```python
from build123d import *

# Parameters (mm, degrees)
ESQUISSE1_W             = 45
ESQUISSE1_H             = 25.2
BOSS_EXTRU_1_DEPTH      = 55
ENL_V_MAT_EXTRU_1_DEPTH = 15.2
ESQUISSE4_W             = 2
ESQUISSE4_H             = 11.757289378
ESQUISSE4_H_2           = 8.71932614
BOSS_EXTRU_2_DEPTH      = 15.2
BOSS_EXTRU_3_DEPTH      = 15.2
CONG_2_R                = 1
CONG_5_R                = 1
CONG_10_R               = 1


with BuildPart() as part:
    # Esquisse1 → Boss.-Extru.1 (new body)
    with BuildSketch(Plane.XY):
        with Locations((0, 2)):
            Rectangle(ESQUISSE1_W, ESQUISSE1_H)
        with BuildLine():
            Line((-4, 3), (-4, -3))
            ThreePointArc((-4, -3), (-6, -5), (-8, -3))
            Line((-8, -3), (-8, 3))
            ThreePointArc((-8, 3), (-6, 5), (-4, 3))
        make_face(mode=Mode.SUBTRACT)
    extrude(amount=BOSS_EXTRU_1_DEPTH)

    # Esquisse3 → Enlèv. mat.-Extru.1 (cut)
    with BuildSketch(Plane.XZ.offset(10.6)):
        with BuildLine():
            Line((5, 55), (5, 39.485421243))
            ThreePointArc((5, 39.485421243), (4.865561607, 38.024962206), (4.46676485, 36.613588609))
            Line((4.46676485, 36.613588609), (0.53323515, 26.386411391))
            ThreePointArc((0.53323515, 26.386411391), (0.134438393, 24.975037794), (0, 23.514578757))
            Line((0, 23.514578757), (0, 0))
            Line((0, 0), (2, 0))
            Line((2, 0), (2, 17.43865228))
            ThreePointArc((2, 17.43865228), (2.100303516, 18.986949278), (2.399537266, 20.509363004))
            Line((2.399537266, 20.509363004), (6.100462734, 34.490636996))
            ThreePointArc((6.100462734, 34.490636996), (6.399696484, 36.013050722), (6.5, 37.56134772))
            Line((6.5, 37.56134772), (6.5, 55))
            Line((6.5, 55), (5, 55))
        make_face()
        with BuildLine():
            Line((5, 17.43865228), (5, 0))
            Line((5, 0), (6.5, 0))
            Line((6.5, 0), (6.5, 15.514578757))
            ThreePointArc((6.5, 15.514578757), (6.634438393, 16.975037794), (7.03323515, 18.386411391))
            Line((7.03323515, 18.386411391), (10.96676485, 28.613588609))
            ThreePointArc((10.96676485, 28.613588609), (11.365561607, 30.024962206), (11.5, 31.485421243))
            Line((11.5, 31.485421243), (11.5, 55))
            Line((11.5, 55), (9.5, 55))
            Line((9.5, 55), (9.5, 37.56134772))
            ThreePointArc((9.5, 37.56134772), (9.399696484, 36.013050722), (9.100462734, 34.490636996))
            Line((9.100462734, 34.490636996), (5.399537266, 20.509363004))
            ThreePointArc((5.399537266, 20.509363004), (5.100303516, 18.986949278), (5, 17.43865228))
        make_face()
    extrude(amount=-ENL_V_MAT_EXTRU_1_DEPTH, mode=Mode.SUBTRACT)

    # Esquisse4 → Boss.-Extru.2 (add)
    with BuildSketch(Plane.XZ.offset(10.6)):
        with Locations((10.5, 49.121355311)):
            Rectangle(ESQUISSE4_W, ESQUISSE4_H)
        with Locations((1, 4.35966307)):
            Rectangle(ESQUISSE4_W, ESQUISSE4_H_2)
    extrude(amount=-BOSS_EXTRU_2_DEPTH)

    # Esquisse5 → Boss.-Extru.3 (add)
    with BuildSketch(Plane.XZ.offset(10.6)):
        with BuildLine():
            Line((5, 53.85), (5, 53.15))
            ThreePointArc((5, 53.15), (5.40348257, 53.21803486), (5.7, 53.5))
            ThreePointArc((5.7, 53.5), (5.40348257, 53.78196514), (5, 53.85))
        make_face()
        with BuildLine():
            Line((5, 51.85), (5, 51.15))
            ThreePointArc((5, 51.15), (5.40348257, 51.21803486), (5.7, 51.5))
            ThreePointArc((5.7, 51.5), (5.40348257, 51.78196514), (5, 51.85))
        make_face()
        with BuildLine():
            Line((5, 49.85), (5, 49.15))
            ThreePointArc((5, 49.15), (5.40348257, 49.21803486), (5.7, 49.5))
            ThreePointArc((5.7, 49.5), (5.40348257, 49.78196514), (5, 49.85))
        make_face()
        with BuildLine():
            Line((5, 47.85), (5, 47.15))
            ThreePointArc((5, 47.15), (5.40348257, 47.21803486), (5.7, 47.5))
            ThreePointArc((5.7, 47.5), (5.40348257, 47.78196514), (5, 47.85))
        make_face()
        with BuildLine():
            Line((5, 45.85), (5, 45.15))
            ThreePointArc((5, 45.15), (5.40348257, 45.21803486), (5.7, 45.5))
            ThreePointArc((5.7, 45.5), (5.40348257, 45.78196514), (5, 45.85))
        make_face()
        with BuildLine():
            Line((5, 43.85), (5, 43.15))
            ThreePointArc((5, 43.15), (5.40348257, 43.21803486), (5.7, 43.5))
            ThreePointArc((5.7, 43.5), (5.40348257, 43.78196514), (5, 43.85))
        make_face()
        with BuildLine():
            Line((5, 41.85), (5, 41.15))
            ThreePointArc((5, 41.15), (5.40348257, 41.21803486), (5.7, 41.5))
            ThreePointArc((5.7, 41.5), (5.40348257, 41.78196514), (5, 41.85))
        make_face()
        with BuildLine():
            Line((5, 39.85), (5, 39.15))
            ThreePointArc((5, 39.15), (5.40348257, 39.21803486), (5.7, 39.5))
            ThreePointArc((5.7, 39.5), (5.40348257, 39.78196514), (5, 39.85))
        make_face()
        with BuildLine():
            Line((5, 1.15), (5, 1.85))
            ThreePointArc((5, 1.85), (5.40348257, 1.78196514), (5.7, 1.5))
            ThreePointArc((5.7, 1.5), (5.40348257, 1.21803486), (5, 1.15))
        make_face()
        with BuildLine():
            Line((5, 15.15), (5, 15.85))
            ThreePointArc((5, 15.85), (5.40348257, 15.78196514), (5.7, 15.5))
            ThreePointArc((5.7, 15.5), (5.40348257, 15.21803486), (5, 15.15))
        make_face()
        with BuildLine():
            Line((5, 13.15), (5, 13.85))
            ThreePointArc((5, 13.85), (5.40348257, 13.78196514), (5.7, 13.5))
            ThreePointArc((5.7, 13.5), (5.40348257, 13.21803486), (5, 13.15))
        make_face()
        with BuildLine():
            Line((5, 11.15), (5, 11.85))
            ThreePointArc((5, 11.85), (5.40348257, 11.78196514), (5.7, 11.5))
            ThreePointArc((5.7, 11.5), (5.40348257, 11.21803486), (5, 11.15))
        make_face()
        with BuildLine():
            Line((5, 9.15), (5, 9.85))
            ThreePointArc((5, 9.85), (5.40348257, 9.78196514), (5.7, 9.5))
            ThreePointArc((5.7, 9.5), (5.40348257, 9.21803486), (5, 9.15))
        make_face()
        with BuildLine():
            Line((5, 7.15), (5, 7.85))
            ThreePointArc((5, 7.85), (5.40348257, 7.78196514), (5.7, 7.5))
            ThreePointArc((5.7, 7.5), (5.40348257, 7.21803486), (5, 7.15))
        make_face()
        with BuildLine():
            Line((5, 5.15), (5, 5.85))
            ThreePointArc((5, 5.85), (5.40348257, 5.78196514), (5.7, 5.5))
            ThreePointArc((5.7, 5.5), (5.40348257, 5.21803486), (5, 5.15))
        make_face()
        with BuildLine():
            Line((5, 3.15), (5, 3.85))
            ThreePointArc((5, 3.85), (5.40348257, 3.78196514), (5.7, 3.5))
            ThreePointArc((5.7, 3.5), (5.40348257, 3.21803486), (5, 3.15))
        make_face()
    extrude(amount=-BOSS_EXTRU_3_DEPTH)

    # Congé2
    cong_2_edges = [part.edges().sort_by_distance(p)[0] for p in [
        (2, -3, 8.71932614),
        (0, -3, 8.71932614),
        (11.5, -3, 43.242710622),
        (9.5, -3, 43.242710622),
    ]]
    fillet(cong_2_edges, radius=CONG_2_R - 0.0001)  # a hair under: the kernel refuses the full size

    # Congé5
    cong_5_edges = [part.edges().sort_by_distance(p)[0] for p in [
        (5, -3, 55),
        (6.5, -3, 55),
        (6.5, -3, 0),
        (5, -3, 0),
    ]]
    fillet(cong_5_edges, radius=CONG_5_R)

    # Congé10
    cong_10_edges = [part.edges().sort_by_distance(p)[0] for p in [
        (-6, 5, 0),
        (-8, 0, 0),
        (-6, -5, 0),
        (-4, 0, 0),
        (-6, 5, 55),
        (-8, 0, 55),
        (-6, -5, 55),
        (-4, 0, 55),
    ]]
    fillet(cong_10_edges, radius=CONG_10_R)


solid = part.part
```
For this review, take the finished solid that the model builds, in its own axes (mm). A direction names the side the tool comes from. Coordinates: 2 decimals unless noted, no trailing zeros. Order: outer loops, then holes, each group sorted by start corner. A loop starts at its lowest first (then second) coordinate and runs counter-clockwise, first axis right, second up. Notation, with made-up numbers: (33, -14.75) -> (53, -14.75) arc R18 ccw to (53, -6.75) -> close; hole circle Ø10 at (53.25, -25). An arc over 180 degrees is marked (long way). Use CSV: the item, a comma, the result in double quotes. Start each with the question number.
Item 1: We need section A-A, the plane x = -6. Give the boundary of the cut face in (y, z).
Item 2: Draft analysis for pull direction X (two halves, no side actions). For faces 1 (the face through (4.224, -3.106, 27.402)), 2 (the face through (0, 2, 0)), state which applies: pulls with the +X half, pulls with the -X half, needs draft (parallel to the pull), parting line crosses it, or undercut.
Item 3: We need section B-B, the plane z = 14.5. Give the boundary of the cut face in (x, y), then the cut area to 3 significant figures.
Item 4: For faces 3 (the face through (-8, 0, 27)), 4 (the face through (5, -3.1, 4.5)), 5 (the face through (6.5, -3, 46)), list the 3-axis set-ups (+Z, -Z, +X, -X, +Y, -Y) from which the entire face can be reached by the end or side of a thin tool; tool diameter is ignored.
Item 5: Wall thickness on probe 1 along X at (y, z) = (3, 21); probe 2 along X at (y, z) = (-4.5, 14.5); probe 3 along X at (y, z) = (-8.75, 38.5): over which ranges is each line inside the solid? List them lowest first.
Item 6: We need section C-C, the plane z = 29.5. Give the boundary of the cut face in (x, y).
Derived:
1,outline,"(-10.6, 0) -> (-6, 0) arc R1 ccw to (-5, 1) -> (-5, 54) arc R1 ccw to (-6, 55) -> (-10.6, 55) -> close; (5, 1) arc R1 ccw to (6, 0) -> (14.6, 0) -> (14.6, 55) -> (6, 55) arc R1 ccw to (5, 54) -> close"
2,face 1,"undercut"
2,face 2,"needs draft"
3,outline,"(-22.5, -10.6) -> (0, -10.6) -> (0, 4.6) -> (2, 4.6) -> (2, -10.6) -> (5, -10.6) -> (5, 4.6) -> (6.5, 4.6) -> (6.5, -10.6) -> (22.5, -10.6) -> (22.5, 14.6) -> (-22.5, 14.6) -> close; hole (-8, -3) arc R2 ccw to (-4, -3) -> (-4, 3) arc R2 ccw to (-8, 3) -> close"
3,area,"1,040 mm^2"
4,face 3,"+Z, -Z"
4,face 4,"-Y"
4,face 5,"+Z, -Y"
5,probe 1,"x = -22.5 to -8, -4 to 0, 2.53 to 5.53, 8.04 to 22.5"
5,probe 2,"x = -22.5 to -7.32, -4.68 to 0, 2 to 5, 6.5 to 22.5"
5,probe 3,"x = -22.5 to 4.94, 6.5 to 9.5, 11.5 to 22.5"
6,outline,"(-22.5, -10.6) -> (1.73, -10.6) -> (1.73, 4.6) -> (4.78, 4.6) -> (4.78, -10.6) -> (7.78, -10.6) -> (7.78, 4.6) -> (11.25, 4.6) -> (11.25, -10.6) -> (22.5, -10.6) -> (22.5, 14.6) -> (-22.5, 14.6) -> close; hole (-8, -3) arc R2 ccw to (-4, -3) -> (-4, 3) arc R2 ccw to (-8, 3) -> close"
